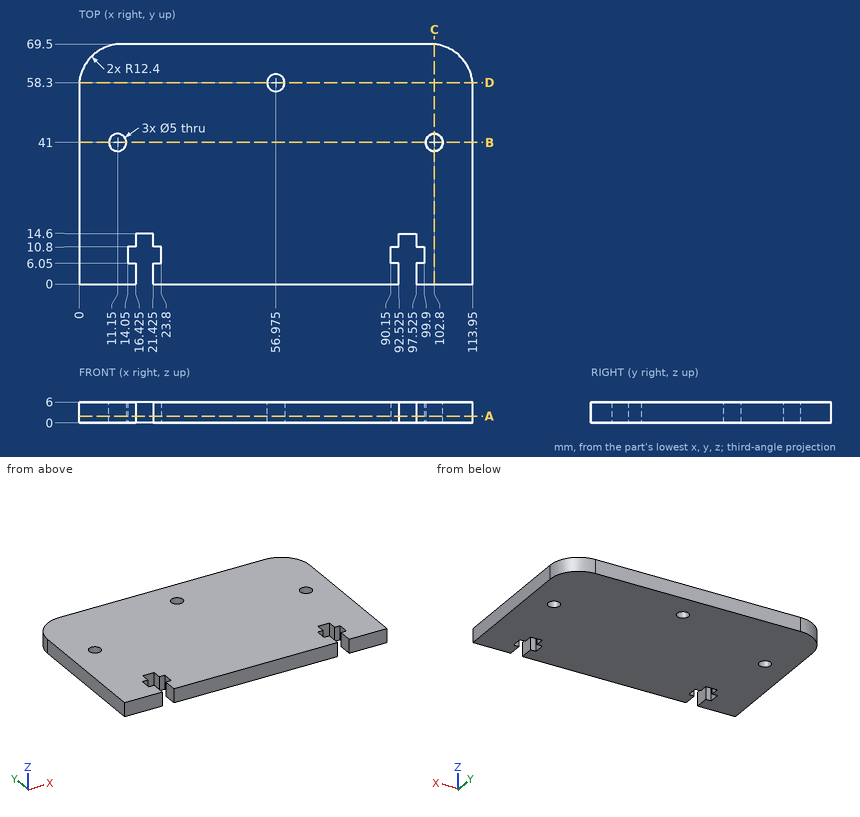
Geometry check sheet. Reference: drawing and pictorial views, mm from the part's lowest x, y, z. Give positions to 0.01 mm unless a question says otherwise; leave off trailing zeros. Order: outer loops, then holes, each group sorted by start corner. A loop starts at its lowest first (then second) coordinate and runs counter-clockwise, first axis right, second up. Notation, with made-up numbers: M 16.25,-40 L 28.25,-40 A19 ccw 28.25,-22 Z; hole C 15.25,6 d1. An arc over 180 degrees is marked long. Answer in a Markdown table with one row per item. Add a question column.
Q1. Sectioned sample at A-A, the plane z = 2. Count the separate pieces of the cut face and the enclosed holes in it, and give its area (3 significant figures).
Q2. Sectioned sample at C-C, the plane x = 102.8. Record the boundary of the cut face in (y, z).
Q3. Thickness scan on L1, parallel to X at y = 39.5, z = 3; L2, parallel to Y at x = 102.8, z = 4.7; L3, parallel to Y at x = 97, z = 5.4. Record the ranges inside material, lowest first.
Q4. Sectioned sample at B-B, the plane y = 41. Record the boundary of the cut face in (x, z).
Q5. Gauge pin test, flat end, axial feed: pin 1 Ø3 at (y, z) = (59.5, 1.5) entering from +X. Record the tip position at first contact, or that the pin passes through.
Q6. Sectioned sample at D-D, the plane y = 58.3. Record the boundary of the cut face in (x, z) (3 decimals), and give its area (3 significant figures).
Verdict:
| question | item | result |
|---|---|---|
| 1 | separate pieces | 1 |
| 1 | enclosed holes | 3 |
| 1 | area | 7,600 mm² |
| 2 | outline | M 0,0 L 38.5,0 L 38.5,6 L 0,6 Z; M 43.5,0 L 69.44,0 L 69.44,6 L 43.5,6 Z |
| 3 | L1 | 0 to 9.15, 13.15 to 100.8, 104.8 to 113.95 |
| 3 | L2 | 0 to 38.5, 43.5 to 69.44 |
| 3 | L3 | 14.6 to 69.5 |
| 4 | outline | M 0,0 L 8.65,0 L 8.65,6 L 0,6 Z; M 13.65,0 L 100.3,0 L 100.3,6 L 13.65,6 Z; M 105.3,0 L 113.95,0 L 113.95,6 L 105.3,6 Z |
| 5 | pin 1 | x = 113.92 |
| 6 | outline | M 0.058,0 L 54.475,0 L 54.475,6 L 0.058,6 Z; M 59.475,0 L 113.892,0 L 113.892,6 L 59.475,6 Z |
| 6 | area | 653 mm² |
